Source: CAD feature listing. Evaluate the final solid. Frame: model axes, mm. A direction names the side the tool comes from. Round coordinates to 2 decimals unless told otherwise and drop trailing zeros. Loops run counter-clockwise (first coordinate to the right, second up) from the corner with the lowest first, then second, coordinate; pieces in that order, holes last. Notation, with made-up numbers: M -30,-17.5 L 27,-17.5 A15 ccw 27,0.5 Z; hole C -29,19.5 d2. An arc over 180 degrees is marked long. Write each question's results on one line, items separated by ' | '. Start each with the question number.
1. Contact query for flat-ended pins moving along their axis: pin 1 Ø0.9 at (y, z) = (-70, 1) entering from -X; pin 2 Ø0.9 at (x, z) = (33.5, 1.5) entering from -Y; pin 3 Ø1.5 at (y, z) = (2, 2) entering from +X. Output: stop coordinate, or through.
2. Section B-B on z = 1.9. Output: boundary loops of the cut face in (x, y), and give its area (3 significant figures).
3. Section D-D on y = -8. Output: boundary loops of the cut face in (x, z), and give its area (3 significant figures).
4. Ray query, line 1 (Y direction, x = 48.5, z = 0.9); line 2 (X direction, y = -65.5, z = 2.6); line 3 (Y direction, x = -17.5, z = 0.55). Return the intervals inside material, ascending.
5. Section C-C on x = 48.5. Output: boundary loops of the cut face in (y, z).
6. Draft query along X for faces 4 (the cylindrical face through (-23.825, -35.964, 1.521)), 5 (the flat face through (-22, -11, 1)), 6 (the flat face through (49, -47, 1)). Return one class per face: released by +X, released by -X, zero draft, split by the parting line, or undercut.
7. Section A-A on x = 37.75. Output: boundary loops of the cut face in (y, z), and give its area (3 significant figures).
8. Set-up query: faces 1 (the flat face through (49, -22, 1)), 2 (the flat face through (36, -69, 1)), 3 (the flat face through (0, -71, 1)). Return all of +Z, -Z, +X, -X, +Y, -Y with unobstructed straight access to the full face (end or side cutting, diameter ignored); none if empty.
Autodesk Inventor part; units mm, degrees
ref_plane "YZ Plane" through (0, 0, 0) normal (1, 0, 0) x (0, 1, 0)
ref_plane "XZ Plane" through (0, 0, 0) normal (0, 1, 0) x (-1, 0, 0)
ref_plane "XY Plane" through (0, 0, 0) normal (0, 0, 1) x (1, 0, 0)
sketch "Sketch1" plane through (0, 0, 0) normal (0, 0, 1) x (1, 0, 0)
  line L0 (0, 3) -> (25, 3)
  line L1 (0, 0) -> (0, 3)
  line L2 (25, 0) -> (25, 3)
  line L3 (25, 0) -> (47, 0)
  line L4 (47, 3) -> (47, -22)
  line L5 (47, -22) -> (50, -22)
  line L6 (50, -22) -> (50, -47)
  line L7 (47, -47) -> (50, -47)
  line L8 (47, -47) -> (47, -72)
  line L9 (25, -69) -> (47, -69)
  line L10 (25, -72) -> (25, -69)
  line L11 (0, -72) -> (25, -72)
  line L12 (0, -72) -> (0, -69)
  line L13 (-22, -69) -> (0, -69)
  line L14 (-22, -47) -> (-22, -72)
  line L15 (-25, -47) -> (-22, -47)
  line L16 (-25, -36) -> (-25, -47)
  line L17 (-25, -22) -> (-22, -22)
  line L18 (-22, 3) -> (-22, -22)
  line L19 (-22, 0) -> (0, 0)
  line L20 (-22, 0) -> (0, 0)
  line L21 (0, 0) -> (0, 3)
  line L22 (0, 3) -> (25, 3)
  line L23 (25, 3) -> (25, 0)
  line L24 (25, 0) -> (47, 0)
  line L25 (47, 0) -> (47, -22)
  line L26 (47, -22) -> (50, -22)
  line L27 (50, -47) -> (50, -22)
  line L28 (50, -47) -> (47, -47)
  line L29 (47, -47) -> (47, -69)
  line L30 (25, -69) -> (47, -69)
  line L31 (25, -69) -> (25, -72)
  line L32 (0, -72) -> (25, -72)
  line L33 (0, -72) -> (0, -69)
  line L34 (0, -69) -> (-22, -69)
  line L35 (-22, -47) -> (-25, -47)
  line L36 (-22, -47) -> (-22, -69)
  line L37 (-25, -47) -> (-25, -36)
  line L38 (-25, -22) -> (-22, -22)
  line L39 (-22, -22) -> (-22, 0)
  line L40 (0, 3) -> (0, 3)
  line L41 (0, 3) -> (0, 0)
  line L42 (25, 0) -> (25, 3)
  line L43 (25, 3) -> (25, 3)
  line L44 (-22, -22) -> (-25, -22)
  line L45 (-25, -22) -> (-25, -36)
extrude "Extrusion1" add sketch "Sketch1" along normal blind 3
sketch "Sketch5" plane through (0, 0, 3) normal (0, 0, 1) x (1, 0, 0)
  line L0 (38.5, -12.7) -> (44.5, -12.7)
  line L1 (0, 0) -> (-22, 0)
  line L2 (-22, -47) -> (-22, -69)
  line L3 (47, -22) -> (47, 0)
  circle A0 centre (48.5, -34.5) radius 1.5
  circle A1 centre (12.5, -70.5) radius 1.5
  circle A2 centre (-23.5, -34.5) radius 1.5
  circle A3 centre (11, 1.5) radius 1.5
  line L4 (25, 0) -> (25, 3)
  line L5 (-22, -22) -> (-25, -22)
  line L6 (-25, -22) -> (-25, -47)
  line L7 (-25, -47) -> (-22, -47)
  line L8 (-22, -69) -> (0, -69)
  line L9 (0, -69) -> (0, -72)
  line L10 (0, -72) -> (25, -72)
  line L11 (25, -72) -> (25, -69)
  line L12 (25, -69) -> (47, -69)
  line L13 (47, -69) -> (47, -47)
  line L14 (47, -47) -> (50, -47)
  line L15 (50, -47) -> (50, -22)
  line L16 (50, -22) -> (47, -22)
  line L17 (47, 0) -> (25, 0)
  line L18 (25, 3) -> (0, 3)
  line L19 (0, 3) -> (0, 0)
  line L20 (-22, 0) -> (-22, -22)
  dimension "d12" = 3
  dimension "d13" = 3
  dimension "d14" = 3
  dimension "d15" = 3
extrude "Extrusion4" cut sketch "Sketch5" against normal blind 25.4 contours A2 | A0
sketch "Sketch6" plane through (0, 0, 3) normal (0, 0, 1) x (1, 0, 0)
  circle A0 centre (37.75, -35.9986) radius 1.5
  point P0 (0, 0)
extrude "Extrusion5" cut sketch "Sketch6" against normal blind 3
sketch "Sketch9" plane through (-25, -47, 0) normal (-1, 0, 0) x (0, 0, 1)
  line L0 (3, 12.5) -> (0, 12.5)
  line L1 (3, 25) -> (3, 12.5)
  line L2 (0, 25) -> (3, 25)
  line L3 (0, 25) -> (0, 12.5)
  line L4 (0, 12.5) -> (0, 0)
  line L5 (0, 0) -> (3, 0)
  line L6 (3, 12.5) -> (3, 0)
  point P0 (0, 47)
extrude "Extrusion8" add sketch "Sketch9" along normal blind 0.5
sketch "Sketch10" plane through (50, -47, 3) normal (1, 0, 0) x (0, 0, -1)
  line L0 (0, 12.5) -> (3, 12.5)
  line L1 (0, 0) -> (0, 12.5)
  line L2 (3, 0) -> (0, 0)
  line L3 (3, 0) -> (3, 12.5)
  line L4 (3, 12.5) -> (3, 25)
  line L5 (3, 25) -> (0, 25)
  line L6 (0, 12.5) -> (0, 25)
  point P0 (3, 47)
extrude "Extrusion9" add sketch "Sketch10" along normal blind 0.5
properties part number "tapa superior"
Taken from the geometry:
1) pin 1: x = 0 | pin 2: y = -69 | pin 3: x = 25
2) outline: M -25.5,-47 L -22,-47 L -22,-69 L 0,-69 L 0,-72 L 25,-72 L 25,-69 L 47,-69 L 47,-47 L 50.5,-47 L 50.5,-22 L 47,-22 L 47,0 L 25,0 L 25,3 L 0,3 L 0,0 L -22,0 L -22,-22 L -25.5,-22 Z; hole C -23.5,-34.5 d3; hole C 37.75,-36 d3; hole C 48.5,-34.5 d3 | area: 5,060 mm^2
3) outline: M -22,0 L 47,0 L 47,3 L -22,3 Z | area: 207 mm^2
4) line 1: -47 to -36, -33 to -22 | line 2: -22 to 47 | line 3: -69 to 0
5) outline: M -47,0 L -36,0 L -36,3 L -47,3 Z; M -33,0 L -22,0 L -22,3 L -33,3 Z
6) face 4: undercut | face 5: released by -X | face 6: zero draft
7) outline: M -69,0 L -37.5,0 L -37.5,3 L -69,3 Z; M -34.5,0 L 0,0 L 0,3 L -34.5,3 Z | area: 198 mm^2
8) face 1: +Z, -Z, +X, +Y | face 2: +Z, -Z, +X, -Y | face 3: +Z, -Z, -X, -Y
